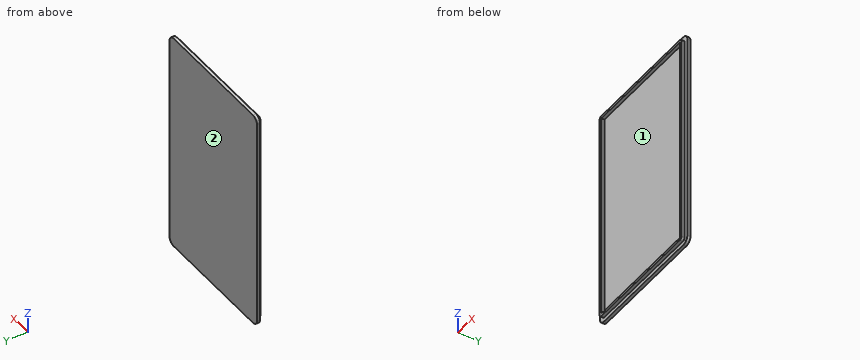
Autodesk Inventor part; units mm, degrees
ref_plane "YZ Plane" through (0, 0, 0) normal (1, 0, 0) x (0, 1, 0)
ref_plane "XZ Plane" through (0, 0, 0) normal (0, 1, 0) x (-1, 0, 0)
ref_plane "XY Plane" through (0, 0, 0) normal (0, 0, 1) x (1, 0, 0)
sketch "Skizze1" plane through (0, 0, 0) normal (0, 1, 0) x (-1, 0, 0)
  line L0 (1, 0) -> (40, 0)
  line L1 (41, 1) -> (41, 70)
  line L2 (40, 71) -> (1, 71)
  line L3 (0, 70) -> (0, 1)
  line L4 (42.2, 70.2) -> (42.2, 0.8)
  line L5 (40.2, -1.2) -> (0.8, -1.2)
  line L6 (-1.2, 0.8) -> (-1.2, 70.2)
  line L7 (0.8, 72.2) -> (40.2, 72.2)
  arc A0 (42.2, 70.2) -> (40.2, 72.2) centre (40.2, 70.2) ccw
  arc A1 (40.2, -1.2) -> (42.2, 0.8) centre (40.2, 0.8) ccw
  arc A2 (-1.2, 0.8) -> (0.8, -1.2) centre (0.8, 0.8) ccw
  arc A3 (0.8, 72.2) -> (-1.2, 70.2) centre (0.8, 70.2) ccw
  arc A4 (41, 70) -> (40, 71) centre (40, 70) ccw
  arc A5 (40, 0) -> (41, 1) centre (40, 1) ccw
  arc A6 (0, 1) -> (1, 0) centre (1, 1) ccw
  arc A7 (1, 71) -> (0, 70) centre (1, 70) ccw
  line L8 (1, 1) -> (1, 70)
  line L9 (1, 70) -> (40, 70)
  line L10 (40, 70) -> (40, 1)
  line L11 (40, 1) -> (1, 1)
  point P0 (0, 0)
  point P1 (41, 71)
  point P2 (41, 0)
  point P3 (0, 71)
  dimension "d0" = 41
  dimension "d1" = 71
  dimension "d2" = 1.2
  dimension "d3" = 2
  dimension "d4" = 1
  dimension "d5" = 1
  dimension "d6" = 1
  dimension "d9" = 1
extrude "Extrusion1" add sketch "Skizze1" along normal blind 1 contours A6 L3 A7 L2 A4 L1 A5 L0 | L4 A1 L5 A2 L6 A3 L7 A0 | L8 L9 L10 L11
extrude "Extrusion2" add sketch "Skizze1" against normal blind 1 contours A6 L3 A7 L2 A4 L1 A5 L0
sketch "Skizze3" plane through (0, -1, 0) normal (0, -1, 0) x (1, 0, 0)
  arc A0 (-41, 1) -> (-40, 0) centre (-40, 1) ccw
  line L0 (-40, 0) -> (-1, 0)
  arc A1 (-1, 0) -> (0, 1) centre (-1, 1) ccw
  line L1 (0, 1) -> (0, 70)
  arc A2 (0, 70) -> (-1, 71) centre (-1, 70) ccw
  line L2 (-1, 71) -> (-40, 71)
  arc A3 (-40, 71) -> (-41, 70) centre (-40, 70) ccw
  line L3 (-41, 70) -> (-41, 1)
  line L4 (-1, 70) -> (-1, 1)
  line L5 (-1, 1) -> (-40, 1)
  line L6 (-40, 1) -> (-40, 70)
  line L7 (-40, 70) -> (-1, 70)
  line L8 (-1, 0.15) -> (-40, 0.15)
  arc A4 (-40.85, 1) -> (-40, 0.15) centre (-40, 1) ccw
  line L9 (-40.85, 1) -> (-40.85, 70)
  arc A5 (-40, 70.85) -> (-40.85, 70) centre (-40, 70) ccw
  line L10 (-40, 70.85) -> (-1, 70.85)
  arc A6 (-0.15, 70) -> (-1, 70.85) centre (-1, 70) ccw
  line L11 (-0.15, 70) -> (-0.15, 1)
  arc A7 (-1, 0.15) -> (-0.15, 1) centre (-1, 1) ccw
  point P0 (0, 0)
  dimension "d12" = 0.15
extrude "Extrusion3" cut sketch "Skizze3" against normal blind 1 contours L3 A3 L2 A2 L1 A1 L0 A0
properties part number "boden"
Read the model definition and answer for the solid it produces. Units are mm, in the model's axes. Face numbers are marked on the shaded views. Round coordinates to 2 decimals unless told otherwise and drop trailing zeros. Write each loop counter-clockwise with the first axis right and the second up, starting at its lowest first coordinate (ties: lowest second). Pieces come first, ordered by that corner, then holes.
1. The part is cut by section A-A, the plane y = -0.6. Determine the outline of the cut face in (x, z).
2. Given pin 1 Ø0.8 at (y, z) = (-0.5, 32) entering from -X; pin 2 Ø13 at (x, z) = (-27, 23.5) entering from -Y; pin 3 Ø0.5 at (x, y) = (-18, -0.5) entering from +Z, each flat-ended and moving along its own axis, determine where each tip first touches the part or whether it passes through.
3. Determine the mould class of the marked faces 1 and 2 for opening direction Z: pulls with the +Z half, pulls with the -Z half, needs draft (parallel to the pull), parting line crosses it, or undercut.
4. The part is cut by section C-C, the plane z = 27.5. Determine the outline of the cut face in (x, y).
5. Straight lines are drawn through the part: L1, parallel to Z at x = -36.5, y = -0.2; L2, parallel to X at y = -0.7, z = 32.5; L3, parallel to Y at x = -33, z = 24.5. For each, find the intervals that lie inside material, in ascending order.
6. The part is cut by section B-B, the plane x = -22. Determine the outline of the cut face in (y, z).
Values:
1. outline: (-40.85, 1) arc R0.85 ccw to (-40, 0.15) - (-1, 0.15) arc R0.85 ccw to (-0.15, 1) - (-0.15, 70) arc R0.85 ccw to (-1, 70.85) - (-40, 70.85) arc R0.85 ccw to (-40.85, 70) - close; hole (-40, 1) - (-1, 1) - (-1, 70) - (-40, 70) - close
2. pin 1: stops at x = -40.85
2. pin 2: stops at y = 0
2. pin 3: stops at z = 70.85
3. face 1: undercut
3. face 2: needs draft
4. outline: (-42.2, 0) - (-40.85, 0) - (-40.85, -1) - (-40, -1) - (-40, 0) - (-1, 0) - (-1, -1) - (-0.15, -1) - (-0.15, 0) - (1.2, 0) - (1.2, 1) - (-42.2, 1) - close
5. L1: z = 0.15 to 1, 70 to 70.85
5. L2: x = -40.85 to -40, -1 to -0.15
5. L3: y = 0 to 1
6. outline: (-1, 0.15) - (0, 0.15) - (0, -1.2) - (1, -1.2) - (1, 72.2) - (0, 72.2) - (0, 70.85) - (-1, 70.85) - (-1, 70) - (0, 70) - (0, 1) - (-1, 1) - close
